Design review of the part built by this model. Coordinates are the model's own, in mm. Face numbers are marked on the shaded views. A direction names the side the tool comes from. Give positions to 0.01 mm unless a question says otherwise; leave off trailing zeros. Write each loop counter-clockwise with the first axis right and the second up, starting at its lowest first coordinate (ties: lowest second). Pieces come first, ordered by that corner, then holes. Notation, with made-up numbers: M 44.25,-39.5 L 91.25,-39.5 A18 ccw 91.25,-23.5 Z; hole C 68,54.25 d7. An arc over 180 degrees is marked long. Answer in a Markdown table with one row per item.
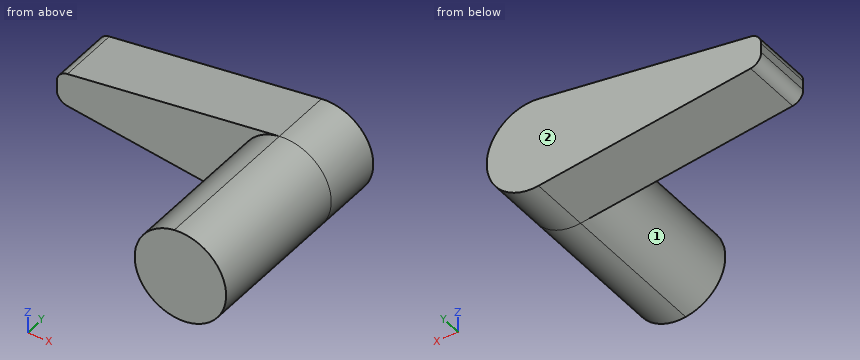
Autodesk Inventor part; units mm, degrees
ref_plane "YZ Plane" through (0, 0, 0) normal (1, 0, 0) x (0, 1, 0)
ref_plane "XZ Plane" through (0, 0, 0) normal (0, 1, 0) x (-1, 0, 0)
ref_plane "XY Plane" through (0, 0, 0) normal (0, 0, 1) x (1, 0, 0)
sketch "Sketch1" plane through (0, 0, 0) normal (0, 1, 0) x (-1, 0, 0)
  circle A0 centre (0, 0) radius 1.5
  line L0 (0.2009, -1.4865) -> (7.5, -0.5)
  line L1 (7.5, 0.5) -> (0.2009, 1.4865)
  line L2 (7.5, 0.5) -> (7.5, -0.5)
  point P0 (7.5, 0)
  dimension "d2" = 3
  dimension "d13" = 7.5
  dimension "d14" = 1
extrude "Extrusion1" add sketch "Sketch1" along normal mid plane 2
sketch "Sketch2" plane through (0, -1, 0) normal (0, 1, 0) x (1, 0, 0)
  arc A0 (-0.2009, -1.4865) -> (-0.2009, 1.4865) centre (0, 0) ccw
  circle A1 centre (0, 0) radius 1.5
extrude "Extrusion2" add sketch "Sketch2" against normal blind 5
fillet "Fillet1" radius 0.4 2 edges at (-7.5, 0, -0.5) (-7.5, 0, 0.5)
properties part number "Pawl2"
1) Add section B-B (y = -4.5). Write out the cut boundary in (x, z), and give its area (3 significant figures).
Geometry says:
| item | result |
|---|---|
| outline | C 0,0 d3 |
| area | 7.07 mm^2 |
2) Add section C-C (x = -1.25). Write out the cut boundary in (y, z), and give its area (3 significant figures).
Geometry says:
| item | result |
|---|---|
| outline | M -6,-0.83 L -1,-0.83 L -1,-1.34 L 1,-1.34 L 1,1.34 L -1,1.34 L -1,0.83 L -6,0.83 Z |
| area | 13.7 mm^2 |
3) For the marked faces 1 and 2, list the 3-axis set-ups (+Z, -Z, +X, -X, +Y, -Y) from which the entire face can be reached by the end or side of a thin tool; tool diameter is ignored.
Geometry says:
| item | result |
|---|---|
| face 1 | -X, -Y |
| face 2 | +Z, -Z, +X, -X, +Y |
4) Add section D-D (z = 1.25). Write out the cut boundary in (x, y).
Geometry says:
| item | result |
|---|---|
| outline | M -1.95,-1 L -0.83,-1 L -0.83,-6 L 0.83,-6 L 0.83,1 L -1.95,1 Z |
5) Add section A-A (z = 0). Write out the cut boundary in (x, y).
Geometry says:
| item | result |
|---|---|
| outline | M -7.5,-1 L -1.5,-1 L -1.5,-6 L 1.5,-6 L 1.5,1 L -7.5,1 Z |
6) To check wall thickness, follow probe 1 along Y at (x, z) = (-3.75, -0.25); probe 2 along X at (y, z) = (-1.5, -0.5); probe 3 along X at (y, z) = (-4.75, -1.1). State the ranges of each line that lie inside material, in increasing order. Write a range as [from, to].
Geometry says:
| item | result |
|---|---|
| probe 1 | [-1, 1] |
| probe 2 | [-1.41, 1.41] |
| probe 3 | [-1.02, 1.02] |
7) Insertion check: P1, Ø1.5, axis at x = -3, z = -0.5, coming from the -Y side; P2, Ø4, axis at x = -4, y = -2, coming from the +Z side. Each pin has a flat end and moves straight along its axis. Give the tip position at first contact, or say it passes through.
Geometry says:
| item | result |
|---|---|
| P1 | y = -1 |
| P2 | z = 1.21 |
